Drawing for the job (mm, zero at the part's lowest x, y, z). A direction names the side the tool comes from. Give positions to 0.01 mm unless a question says otherwise; leave off trailing zeros. Write each loop counter-clockwise with the first axis right and the second up, starting at its lowest first coordinate (ties: lowest second). Pieces come first, ordered by that corner, then holes.
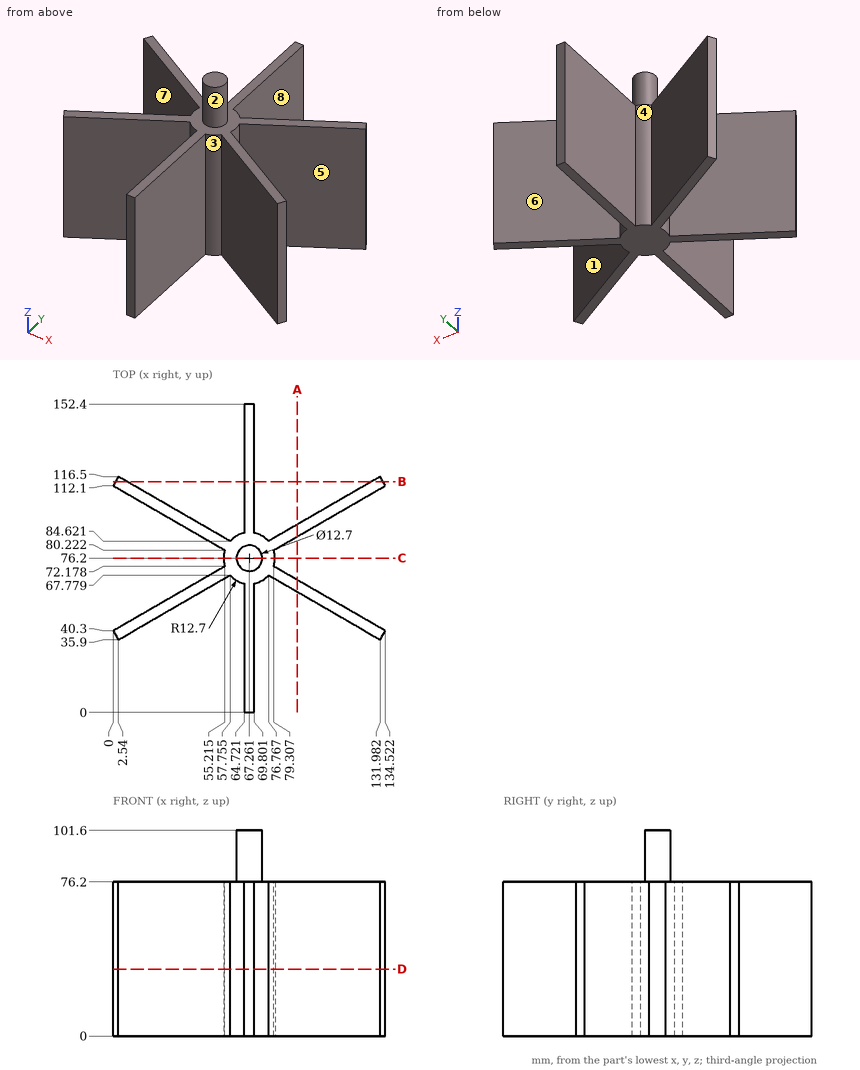
1. Which spindle directions (+Z, -Z, +X, -X, +Y, -Y) get a long thin tool onto all of the face, cutting with end or side? Do the marked faces 1, 2, 3 and 4. Say none if no direction does.
Calculated:
face 1: +Z, -Z, +X
face 2: +Z
face 3: +Z, -Z, -Y
face 4: +Z, -Z, +Y
2. Slice it at D-D, the plane z = 33. Write the cut outline in (x, y) (1 decimal).
Calculated:
outline: (0, 40.3) - (2.5, 35.9) - (57.8, 67.8) arc R12.7 ccw to (64.7, 63.8) - (64.7, 0) - (69.8, 0) - (69.8, 63.8) arc R12.7 ccw to (76.8, 67.8) - (132, 35.9) - (134.5, 40.3) - (79.3, 72.2) arc R12.7 ccw to (79.3, 80.2) - (134.5, 112.1) - (132, 116.5) - (76.8, 84.6) arc R12.7 ccw to (69.8, 88.6) - (69.8, 152.4) - (64.7, 152.4) - (64.7, 88.6) arc R12.7 ccw to (57.8, 84.6) - (2.5, 116.5) - (0, 112.1) - (55.2, 80.2) arc R12.7 ccw to (55.2, 72.2) - close
3. Slice it at A-A, the plane x = 91. Write the cut outline in (y, z).
Calculated:
outline: (59.56, 0) - (65.43, 0) - (65.43, 76.2) - (59.56, 76.2) - close; (86.97, 0) - (92.84, 0) - (92.84, 76.2) - (86.97, 76.2) - close
4. Pin check, flat tips, straight feed: P1, Ø1, axis at y = 124.5, z = 37.5, coming from the -X side; P2, Ø10, axis at y = 102.5, z = 46, coming from the +X side (1 decimal); P3, Ø3, axis at x = 117.5, z = 59, coming from the -Y side (1 decimal). Stop position of each tip, or through.
Calculated:
P1: stops at x = 64.72
P2: stops at x = 126.6
P3: stops at y = 43.4
5. Probe probe 1 along X at (y, z) = (46.5, 71.5) (1 decimal); probe 2 along X at (y, z) = (12.5, 71.5); probe 3 along Y at (x, z) = (13.5, 4) (1 decimal). List the from-to ranges inside material, lowest first.
Calculated:
probe 1: x = 10.7 to 20.9, 64.7 to 69.8, 113.6 to 123.8
probe 2: x = 64.72 to 69.8
probe 3: y = 42.2 to 48.1, 104.3 to 110.2
6. Slice it at C-C, the plane y = 76.2. Write the cut outline in (x, z).
Calculated:
outline: (54.56, 0) - (79.96, 0) - (79.96, 76.2) - (73.61, 76.2) - (73.61, 101.6) - (60.91, 101.6) - (60.91, 76.2) - (54.56, 76.2) - close
7. Pull direction X, two halves, no side cores. Call the marked faces 5, 6, 7 and 8: +X half, -X half, draft (parallel to the pull), parting line (faces both ways), or undercut.
Calculated:
face 5: +X half
face 6: undercut
face 7: -X half
face 8: undercut
8. Slice it at B-B, the plane y = 114. Write the cut outline in (x, z) (1 decimal), and give its area (3 significant figures).
Calculated:
outline: (1.1, 0) - (6.9, 0) - (6.9, 76.2) - (1.1, 76.2) - close; (64.7, 0) - (69.8, 0) - (69.8, 76.2) - (64.7, 76.2) - close; (127.7, 0) - (133.4, 0) - (133.4, 76.2) - (127.7, 76.2) - close
area: 1,270 mm2
